Work out the finished part from the listing and answer in its coordinate system (mm). Give positions to 0.01 mm unless a question says otherwise; leave off trailing zeros. Order: outer loops, then holes, each group sorted by start corner. A loop starts at its lowest first (then second) coordinate and runs counter-clockwise, first axis right, second up. Notation, with made-up numbers: (58.5, -21) - (115.5, -21) arc R36 ccw to (115.5, 16) - close; hole circle Ø3 at (78, -28.5). An arc over 180 degrees is marked (long way). Put each result on its own line as item: value.
```python
from build123d import *

# Parameters (mm, degrees)
SKETCH018_W           = 510
SKETCH018_H           = 350
PAD015_DEPTH          = 5
SKETCH019_R           = 8
SKETCH019_R_2         = 4.25
POCKET011_DEPTH       = 5.001
FILLET005_R           = 20
SKETCH020_R           = 2
POCKET012_DEPTH       = 5.001
CHAMFER009_SIZE       = 6
CHAMFER010_SIZE       = 0.1
CHAMFER011_SIZE       = 0.1
SKETCH052_W           = 45
SKETCH052_H           = 10
POCKET033_DEPTH       = 5.001
CHAMFER024_SIZE       = 2.99
SKETCH068_R           = 2.5
POCKET043_DEPTH       = 5.001
CLONE_PLACEMENT_ANGLE = 90


with BuildPart() as part:
    # Sketch018 → Pad015 (new body)
    with BuildSketch(Plane.XY):
        with Locations((-20, 41.2)):
            Rectangle(SKETCH018_W, SKETCH018_H)
    extrude(amount=PAD015_DEPTH)

    # Sketch019 (on Face6 of Pad015) → Pocket011 (cut, through all)
    with BuildSketch(Plane.XY.offset(5)):
        with Locations((-238, 0)):
            Circle(SKETCH019_R)
        with Locations((225, 0)):
            Circle(SKETCH019_R_2)
        with BuildLine():
            ThreePointArc((-164.573184, 24.404903), (-159.323184, 19.154903), (-154.073184, 24.404903))
            Line((-154.073184, 24.404903), (-154.073184, 216.2))
            ThreePointArc((-154.073184, 216.2), (-159.323184, 221.45), (-164.573184, 216.2))
            Line((-164.573184, 24.404903), (-164.573184, 216.2))
        make_face()
        with BuildLine():
            ThreePointArc((-74.573184, -36.417713), (-69.323184, -41.667713), (-64.073184, -36.417713))
            Line((-64.073184, -36.417713), (-64.073184, 216.2))
            ThreePointArc((-64.073184, 216.2), (-69.323184, 221.45), (-74.573184, 216.2))
            Line((-74.573184, -36.417713), (-74.573184, 216.2))
        make_face()
        with BuildLine():
            ThreePointArc((15.426816, 28.977719), (20.676816, 23.727719), (25.926816, 28.977719))
            Line((25.926816, 28.977719), (25.926816, 216.2))
            ThreePointArc((25.926816, 216.2), (20.676816, 221.45), (15.426816, 216.2))
            Line((15.426816, 28.977719), (15.426816, 216.2))
        make_face()
        with BuildLine():
            ThreePointArc((105.426816, 89.800335), (110.676816, 84.550335), (115.926816, 89.800335))
            Line((115.926816, 89.800335), (115.926816, 216.2))
            ThreePointArc((115.926816, 216.2), (110.676816, 221.45), (105.426816, 216.2))
            Line((105.426816, 89.800335), (105.426816, 216.2))
        make_face()
    extrude(amount=-POCKET011_DEPTH, mode=Mode.SUBTRACT)

    # Fillet005
    fillet005_edges = [part.edges().sort_by_distance(p)[0] for p in [
        (-275, 216.2, 2.5),
        (-275, -133.8, 2.5),
    ]]
    fillet(fillet005_edges, radius=FILLET005_R)

    # Sketch020 (on Face5 of Fillet005) → Pocket012 (cut, through all)
    with BuildSketch(Plane.XY.offset(5)):
        with Locations((-255, 196.2)):
            Circle(SKETCH020_R)
        with Locations((-255, -113.8)):
            Circle(SKETCH020_R)
        with Locations((215, -113.8)):
            Circle(SKETCH020_R)
        with Locations((215, 196.2)):
            Circle(SKETCH020_R)
    extrude(amount=-POCKET012_DEPTH, mode=Mode.SUBTRACT)

    # Chamfer009
    chamfer009_edges = [part.edges().sort_by_distance(p)[0] for p in [
        (-164.573184, 216.2, 2.5),
        (-154.073184, 216.2, 2.5),
        (-74.573184, 216.2, 2.5),
        (-64.073184, 216.2, 2.5),
        (15.426816, 216.2, 2.5),
        (25.926816, 216.2, 2.5),
        (105.426816, 216.2, 2.5),
        (115.926816, 216.2, 2.5),
    ]]
    chamfer(chamfer009_edges, length=CHAMFER009_SIZE)

    # Chamfer010
    chamfer010_edges = [part.edges().sort_by_distance(p)[0] for p in [
        (-212.786592, 216.2, 5),
        (-114.323184, 216.2, 5),
        (-24.323184, 216.2, 5),
        (65.676816, 216.2, 5),
        (178.463408, 216.2, 5),
    ]]
    chamfer(chamfer010_edges, length=CHAMFER010_SIZE)

    # Chamfer011
    chamfer011_edges = [part.edges().sort_by_distance(p)[0] for p in [
        (-257, 196.2, 5),
        (-257, -113.8, 5),
        (213, -113.8, 5),
        (213, 196.2, 5),
    ]]
    chamfer(chamfer011_edges, length=CHAMFER011_SIZE)

    # Sketch052 (on Face1 of Chamfer011) → Pocket033 (cut, through all)
    with BuildSketch(Plane.XY.offset(5)):
        with Locations((-173.573184, 211.2)):
            Rectangle(SKETCH052_W, SKETCH052_H)
        with Locations((-83.573184, 211.2)):
            Rectangle(SKETCH052_W, SKETCH052_H)
        with Locations((6.426816, 211.2)):
            Rectangle(SKETCH052_W, SKETCH052_H)
        with Locations((96.426816, 211.2)):
            Rectangle(SKETCH052_W, SKETCH052_H)
    extrude(amount=-POCKET033_DEPTH, mode=Mode.SUBTRACT)

    # Chamfer024
    chamfer024_edges = [part.edges().sort_by_distance(p)[0] for p in [
        (-164.573184, 206.2, 2.5),
        (-154.073184, 206.2, 2.5),
        (-74.573184, 206.2, 2.5),
        (-64.073184, 206.2, 2.5),
        (15.426816, 206.2, 2.5),
        (25.926816, 206.2, 2.5),
        (105.426816, 206.2, 2.5),
        (115.926816, 206.2, 2.5),
    ]]
    chamfer(chamfer024_edges, length=CHAMFER024_SIZE)

    # Sketch068 (on Face1 of Chamfer024) → Pocket043 (cut, through all)
    with BuildSketch(Plane.XY.offset(5)):
        with Locations((-217.5, -77)):
            Circle(SKETCH068_R)
        with Locations((-217.5, -121)):
            Circle(SKETCH068_R)
    extrude(amount=-POCKET043_DEPTH, mode=Mode.SUBTRACT)


with BuildPart() as part_1:
    # Body011 placement: moved
    add(part.part.moved(Location((0, 0, 10.25))))


with BuildPart() as part_2:
    # Clone placement: moved
    add(part_1.part.moved(Location((216.2, 275, -15.25))).rotate(Axis((216.2, 275, -15.25), (0, 0, 1)), CLONE_PLACEMENT_ANGLE))


solid = part_2.part
```
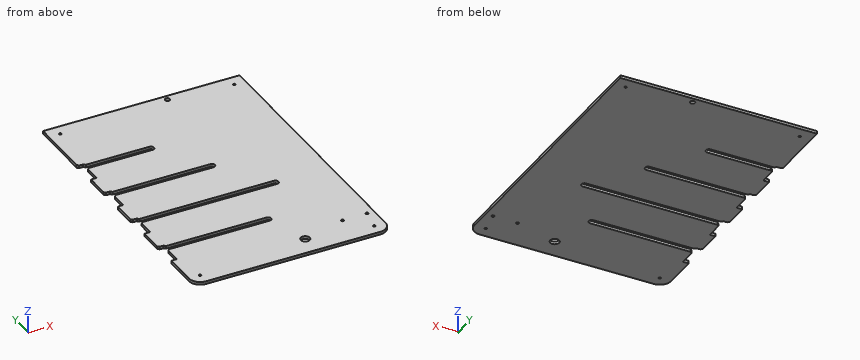
(1) Straight lines are drawn through the part: line 1 (X direction, y = 57.5, z = -2.2); line 2 (Y direction, x = 40, z = -0.8); line 3 (X direction, y = 490, z = -2.3). For each, find the intervals that lie inside material, in ascending order.
Geometry check:
line 1: x = 0 to 290.7, 295.7 to 334.7, 339.7 to 350
line 2: y = 0 to 110.43, 120.93 to 200.43, 210.93 to 290.43, 300.93 to 380.43, 390.93 to 510
line 3: x = 0 to 18, 22 to 328, 332 to 350
(2) Section B-B, the plane x = 72.5 is taken. Write down the section's boundary in (y, z).
Geometry check:
outline: (0, -5) - (110.43, -5) - (110.43, 0) - (0.1, 0) - (0, -0.1) - close; (120.93, -5) - (200.43, -5) - (200.43, 0) - (120.93, 0) - close; (210.93, -5) - (290.43, -5) - (290.43, 0) - (210.93, 0) - close; (300.93, -5) - (380.43, -5) - (380.43, 0) - (300.93, 0) - close; (390.93, -5) - (510, -5) - (510, 0) - (390.93, 0) - close
(3) Section A-A, the plane x = 237 is taken. Write down the section's boundary in (y, z), then the cut area to 3 significant figures.
Geometry check:
outline: (0, -5) - (200.43, -5) - (200.43, 0) - (0.1, 0) - (0, -0.1) - close; (210.93, -5) - (510, -5) - (510, 0) - (210.93, 0) - close
area: 2,500 mm²
(4) Given pin 1 (1.5 mm diameter, centred on x = 5, z = -1.5, fed in from -Y), flat-ended and moving along its own axis, determine where the tip first touches the part or whether it passes through.
Geometry check:
pin 1: stops at y = 5.97
(5) Section C-C, the plane z = -4 is taken. Count the separate pieces of the cut face and the enclosed holes in it, then the cut area to 3 significant figures.
Geometry check:
separate pieces: 1
enclosed holes: 8
area: 168,000 mm²
